from build123d import *

# Parameters (mm, degrees)
SKETCH1_W           = 10
SKETCH1_H           = 3.105775443
BOSS_EXTRUDE1_DEPTH = 15.14
FILLET1_R           = 0.5


with BuildPart() as part:
    # Sketch1 → Boss-Extrude1 (new body)
    with BuildSketch(Plane.XY):
        with Locations((-0.008293574, -2.2925e-05)):
            Rectangle(SKETCH1_W, SKETCH1_H)
    extrude(amount=BOSS_EXTRUDE1_DEPTH)

    # Loft1: read off the stored shape, not the designer's step
    # Loft1: loft between two sections, ruled curve by curve
    loft1_from = [
        Edge.make_bspline([(6.002368105, 5, 15.14), (4.973125798, 5, 15.14), (3.004819926, 5, 15.14), (0.185859297, 5, 15.14), (-2.58508535, 5, 15.14), (-4.44969412, 5, 15.14), (-5.449891462, 5, 15.14), (-5.57771544, 5, 15.14), (-5.783318565, 5, 15.14), (-5.907849178, 5, 15.14), (-5.972093141, 5, 15.14), (-6.17467612, 5, 15.14), (-6.499597583, 4.964301348, 15.14), (-6.934896014, 4.832707278, 15.14), (-7.32552261, 4.634429877, 15.14), (-7.673911431, 4.373864242, 15.14), (-7.978763997, 4.050324082, 15.14), (-8.234306918, 3.655920908, 15.14), (-8.396723796, 3.254240148, 15.14), (-8.480332717, 2.862623296, 15.14), (-8.5, 2.631885527, 15.14), (-8.5, 2.075292876, 15.14), (-8.5, 1.127457579, 15.14), (-8.5, -0.819864409, 15.14), (-8.5, -3.191164425, 15.14), (-8.5, -4.454054832, 15.14), (-8.5, -5, 15.14)], [0, 0, 0, 0, 0.111510841, 0.223021681, 0.334532522, 0.446043363, 0.446043363, 0.451912354, 0.457781346, 0.463650337, 0.469519329, 0.469519329, 0.506254839, 0.54299035, 0.57972586, 0.61646137, 0.653196881, 0.689932391, 0.726667901, 0.745035656, 0.763403412, 0.763403412, 0.822552559, 0.881701706, 0.940850853, 1, 1, 1, 1], 3),
        Edge.make_bspline([(8.5, -5, 15.14), (8.500991996, -4.575244993, 15.14), (8.503176578, -3.63984652, 15.14), (8.508751194, -1.252896386, 15.14), (8.51432581, 1.134053748, 15.14), (8.516510392, 2.069452221, 15.14), (8.517811111, 2.626396957, 15.14), (8.49908527, 2.846946207, 15.14), (8.443489244, 3.123561182, 15.14), (8.367638554, 3.363722111, 15.14), (8.245865367, 3.65118142, 15.14), (8.059926267, 3.961930691, 15.14), (7.790063704, 4.279208373, 15.14), (7.471784056, 4.547888472, 15.14), (7.160345054, 4.732669981, 15.14), (6.872434615, 4.853372684, 15.14), (6.631993106, 4.928329205, 15.14), (6.355173173, 4.982895557, 15.14), (6.13455577, 5.000800601, 15.14), (6.002368105, 5, 15.14)], [0, 0, 0, 0, 0.111365706, 0.222731413, 0.334097119, 0.445462826, 0.445462826, 0.480121399, 0.514779973, 0.549438546, 0.584097119, 0.653414266, 0.722731413, 0.79204856, 0.861365706, 0.89602428, 0.930682853, 0.965341427, 1, 1, 1, 1], 3),
        Edge.make_line((-8.5, -5, 15.14), (8.5, -5, 15.14)),
    ]
    loft1_to = [
        Edge.make_bspline([(1.898763427, -2, 55.14), (1.68912791, -2, 55.14), (1.247791237, -2, 55.14), (0.527731018, -2, 55.14), (-0.222420428, -2, 55.14), (-0.713736573, -2, 55.14), (-0.963736573, -2, 55.14), (-0.986728567, -2, 55.14), (-1.019071695, -2, 55.14), (-1.054765163, -2, 55.14), (-1.080945918, -2, 55.14), (-1.228240938, -2, 55.14), (-1.496918662, -2.025435314, 55.14), (-1.911785618, -2.15285696, 55.14), (-2.306346344, -2.382510015, 55.14), (-2.62960532, -2.68644458, 55.14), (-2.864851797, -3.028969372, 55.14), (-3.011847525, -3.375243405, 55.14), (-3.075118823, -3.64816943, 55.14), (-3.0978707, -3.853987875, 55.14), (-3.101236573, -3.952199478, 55.14), (-3.101236573, -4.153930631, 55.14), (-3.101236573, -4.297062563, 55.14), (-3.101236573, -4.527630405, 55.14), (-3.101236573, -4.731947482, 55.14), (-3.101236573, -4.888802183, 55.14), (-3.101236573, -5, 55.14)], [0, 0, 0, 0, 0.111510841, 0.223021681, 0.334532522, 0.446043363, 0.446043363, 0.451912354, 0.457781346, 0.463650337, 0.469519329, 0.469519329, 0.506254839, 0.54299035, 0.57972586, 0.61646137, 0.653196881, 0.689932391, 0.726667901, 0.745035656, 0.763403412, 0.763403412, 0.822552559, 0.881701706, 0.940850853, 1, 1, 1, 1], 3),
        Edge.make_bspline([(3.898763427, -5, 55.14), (3.898763427, -4.846256203, 55.14), (3.898763427, -4.714582876, 55.14), (3.898763427, -4.5, 55.14), (3.898763427, -4.285417124, 55.14), (3.898763427, -4.153743797, 55.14), (3.898763427, -3.952152769, 55.14), (3.895391319, -3.852913488, 55.14), (3.877383526, -3.693016744, 55.14), (3.843592793, -3.521678819, 55.14), (3.772300297, -3.279550251, 55.14), (3.62424883, -2.954199991, 55.14), (3.327418957, -2.571379789, 55.14), (2.944616956, -2.274539085, 55.14), (2.619245408, -2.126493121, 55.14), (2.377114625, -2.05518085, 55.14), (2.20577222, -2.021376458, 55.14), (2.045857954, -2.003369443, 55.14), (1.946610658, -2, 55.14), (1.898763427, -2, 55.14)], [0, 0, 0, 0, 0.111365706, 0.222731413, 0.334097119, 0.445462826, 0.445462826, 0.480121399, 0.514779973, 0.549438546, 0.584097119, 0.653414266, 0.722731413, 0.79204856, 0.861365706, 0.89602428, 0.930682853, 0.965341427, 1, 1, 1, 1], 3),
        Edge.make_line((-3.101236573, -5, 55.14), (3.898763427, -5, 55.14)),
    ]
    loft1 = Solid(Shell([*[Face.make_surface_from_curves(loft1_from[k], loft1_to[k]) for k in range(3)], Face(Wire(loft1_from)), Face(Wire(loft1_to))]))
    add(loft1)

    # Fillet1
    fillet1_edges = [part.edges().sort_by_distance(p)[0] for p in [
        (-5.008293574, 1.552864796, 7.57),
        (4.991706426, 1.552864796, 7.57),
    ]]
    fillet(fillet1_edges, radius=FILLET1_R)


solid = part.part
Build history of the part. All positions in model axes, mm. A direction names the side the tool comes from. Round coordinates to 2 decimals unless told otherwise and drop trailing zeros. Write each loop counter-clockwise with the first axis right and the second up, starting at its lowest first coordinate (ties: lowest second). Pieces come first, ordered by that corner, then holes. Notation, with made-up numbers: M -7,35.5 L 8,35.5 A31 cw 8,73.5 Z; hole C 12,-26.75 d9. An arc over 180 degrees is marked long. Answer as a JSON object with one key per item and string values. Group by question number.
(1) Flat gauge pins, fed straight in: pin 1 (1.3 mm diameter, centred on y = -0.5, z = 10.5, fed in from -X); pin 2 (1 mm diameter, centred on y = 2, z = 30, fed in from +X); pin 3 (3 mm diameter, centred on x = -1.5, y = 0, fed in from -Z); pin 4 (2.5 mm diameter, centred on x = -2, z = 8.5, fed in from +Y). Where does each tip first touch, or does it go through?
(2) Which spindle directions (+Z, -Z, +X, -X, +Y, -Y) get a long thin tool onto all of the face, cutting with end or side? Do faces 1 (the flat face through (-5.008, 0, 7)), 2 (the flat face through (4.992, 0, 7)), 3 (the flat face through (0, 1.553, 7)), 4 (the flat face through (0, -1.553, 7)), 5 (the flat face through (0, -3, 55.14)). Say none if no direction does.
(3) Cut at A-A (z = 11). Give the cut face in (x, y), and give its area (3 significant figures).
(4) Drill centre lines: L1, parallel to Y at x = -3.5, z = 15; L2, parallel to Z at x = -1.75, y = -3.5; L3, parallel to Y at x = 1, z = 22. Where is each one in solid material? Low to high.
Responses:
{
 "1": {"pin 1": "stops at x = -5.01", "pin 2": "stops at x = 6.34", "pin 3": "stops at z = 0", "pin 4": "stops at y = 1.55"},
 "2": {"face 1": "-Z, -X, +Y, -Y", "face 2": "-Z, +X, +Y, -Y", "face 3": "-Z, +X, -X, +Y", "face 4": "-Z, +X, -X, -Y", "face 5": "+Z, +X, -X, +Y, -Y"},
 "3": {"outline": "M -5.01,-1.55 L 4.99,-1.55 L 4.99,1.05 A0.5 ccw 4.49,1.55 L -4.51,1.55 A0.5 ccw -5.01,1.05 Z", "area": "31.0 mm2"},
 "4": {"L1": "y = -1.55 to 1.55", "L2": "z = 15.14 to 55.14", "L3": "y = -5 to 3.8"}
}
